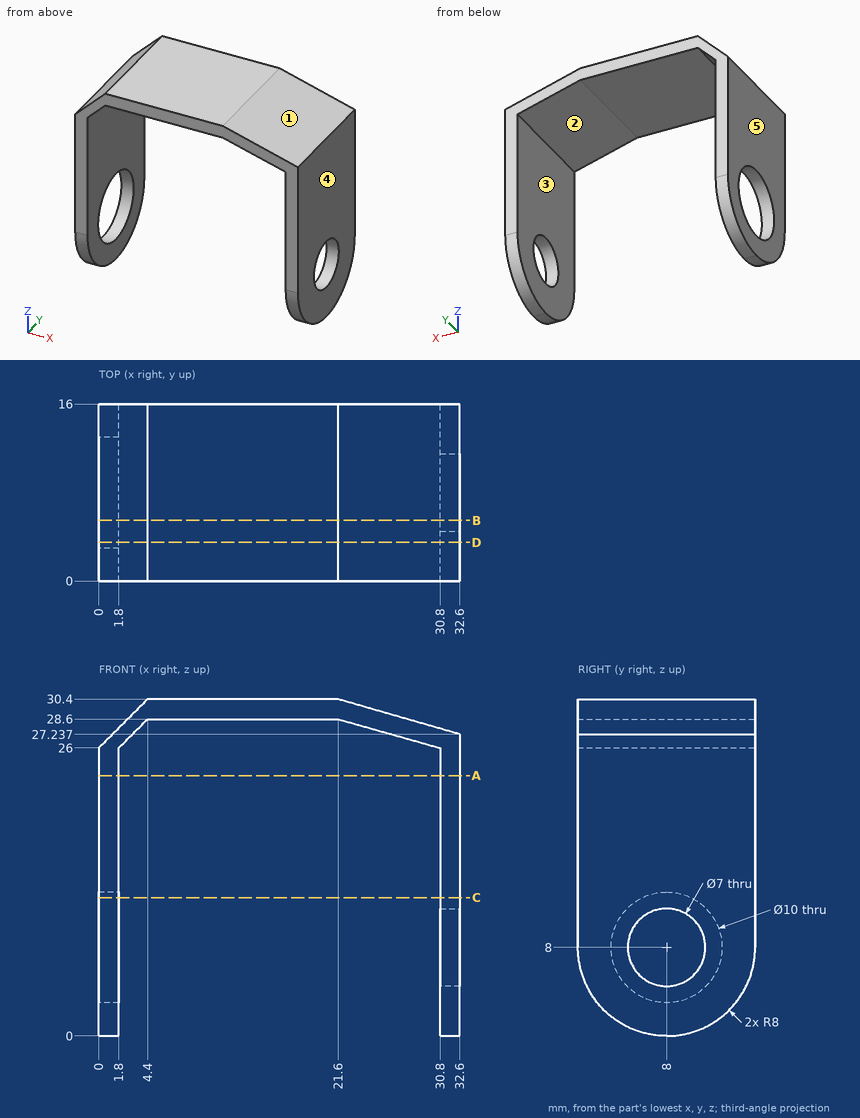
Answer from the drawing. Dimensions are ordinates in mm from the lowest x, y and z of the part. A direction names the side the tool comes from. Round coordinates to 2 decimals unless told otherwise and drop trailing zeros. Write each loop counter-clockwise with the first axis right and the second up, starting at its lowest first coordinate (ties: lowest second). Pieces come first, ordered by that corner, then holes. Notation, with made-up numbers: (82, -11) - (91, -11) arc R33 ccw to (91, 27) - close; hole circle Ø10 at (85.5, 0.5). An arc over 180 degrees is marked (long way). Use a Markdown table: item, result.
(1) The part is cut by section D-D (y = 3.5). Write down the section's boundary in (x, z) (1 decimal), then the cut area to 3 significant figures.
Reported:
| item | result |
|---|---|
| outline | (0, 1.4) - (1.8, 1.4) - (1.8, 5.8) - (0, 5.8) - close; (0, 10.2) - (1.8, 10.2) - (1.8, 26) - (4.4, 28.6) - (21.6, 28.6) - (30.8, 26) - (30.8, 1.4) - (32.6, 1.4) - (32.6, 27.2) - (21.6, 30.4) - (4.4, 30.4) - (0, 26) - close |
| area | 137 mm2 |
(2) Straight lines are drawn through the part: line 1 along Y through (x, z) = (31, 8); line 2 along Y through (x, z) = (0.4, 8); line 3 along X through (y, z) = (7.75, 20.5). For each, find the intervals that lie inside material, in ascending order. Write a range as [from, to].
Reported:
| item | result |
|---|---|
| line 1 | [0, 4.5], [11.5, 16] |
| line 2 | [0, 3], [13, 16] |
| line 3 | [0, 1.8], [30.8, 32.6] |
(3) The part is cut by section C-C (z = 12.5). Write down the section's boundary in (x, y).
Reported:
| item | result |
|---|---|
| outline | (0, 0) - (1.8, 0) - (1.8, 5.82) - (0, 5.82) - close; (0, 10.18) - (1.8, 10.18) - (1.8, 16) - (0, 16) - close; (30.8, 0) - (32.6, 0) - (32.6, 16) - (30.8, 16) - close |
(4) The mould has two halves that part along X. Classify the marked faces 3, 4 and 5: released by +X, released by -X, zero draft, split by the parting line, or undercut.
Reported:
| item | result |
|---|---|
| face 3 | undercut |
| face 4 | released by +X |
| face 5 | released by -X |
(5) The part is cut by section B-B (y = 5.5). Write down the section's boundary in (x, z), then the cut area to 3 significant figures.
Reported:
| item | result |
|---|---|
| outline | (0, 0.4) - (1.8, 0.4) - (1.8, 3.67) - (0, 3.67) - close; (0, 12.33) - (1.8, 12.33) - (1.8, 26) - (4.4, 28.6) - (21.6, 28.6) - (30.8, 26) - (30.8, 10.45) - (32.6, 10.45) - (32.6, 27.24) - (21.6, 30.4) - (4.4, 30.4) - (0, 26) - close; (30.8, 0.4) - (32.6, 0.4) - (32.6, 5.55) - (30.8, 5.55) - close |
| area | 124 mm2 |
(6) The part is cut by section A-A (z = 23.5). Write down the section's boundary in (x, y).
Reported:
| item | result |
|---|---|
| outline | (0, 0) - (1.8, 0) - (1.8, 16) - (0, 16) - close; (30.8, 0) - (32.6, 0) - (32.6, 16) - (30.8, 16) - close |
(7) This flat-tipped pin is pushed along its axis until it touches: pin 1 Ø4 at (x, y) = (26.5, 9.5) entering from -Z. Where does it stop, or does it pass through?
Reported:
| item | result |
|---|---|
| pin 1 | z = 26.65 |
(8) Which of the six approach directions +Z, -Z, +X, -X, +Y, -Y give full straight-line access (tool end or side, diameter ignored) to the marked faces 1 and 2?
Reported:
| item | result |
|---|---|
| face 1 | +Z, +X, +Y, -Y |
| face 2 | -Z, +Y, -Y |
